Autodesk Inventor part; units mm, degrees
ref_plane "YZ Plane" through (0, 0, 0) normal (1, 0, 0) x (0, 1, 0)
ref_plane "XZ Plane" through (0, 0, 0) normal (0, 1, 0) x (-1, 0, 0)
ref_plane "XY Plane" through (0, 0, 0) normal (0, 0, 1) x (1, 0, 0)
sketch "Sketch1" plane through (0, 0, 0) normal (0, 1, 0) x (-1, 0, 0)
  line L0 (10, 67.88) -> (-10, 67.88)
  line L1 (-10, 67.88) -> (-10, -10)
  line L2 (-10, -10) -> (10, -10)
  line L3 (10, -10) -> (10, 67.88)
  point P0 (0, 0)
  dimension "d0" = 20
  dimension "d1" = 77.88
extrude "Extrusion1" add sketch "Sketch1" along normal blind 2
sketch "Sketch2" plane through (0, 2, 0) normal (0, 1, 0) x (1, 0, 0)
  line L0 (-10, -67.88) -> (10, -67.88)
  line L1 (0, -67.88) -> (-6.35, -67.88)
  line L2 (-6.35, -56.98) -> (6.35, -56.98)
  line L3 (6.35, -67.88) -> (0, -67.88)
  line L4 (10, 10) -> (-10, 10)
  line L5 (-6.35, -0.9) -> (6.35, -0.9)
  line L6 (-6.35, 10) -> (6.35, 10)
  line L7 (-6.35, -67.88) -> (-10, -67.88)
  line L8 (-10, 10) -> (-10, -67.88)
  line L9 (-10, -56.98) -> (-6.35, -56.98)
  line L10 (6.35, -67.88) -> (10, -67.88)
  line L11 (10, -67.88) -> (10, 10)
  line L12 (10, -56.98) -> (6.35, -56.98)
  line L13 (6.35, -0.9) -> (10, -0.9)
  line L14 (10, 10) -> (6.35, 10)
  line L15 (10, -0.9) -> (10, 10)
  line L16 (10, -67.88) -> (10, -56.98)
  line L17 (-10, -67.88) -> (-10, -56.98)
  line L18 (-6.35, -0.9) -> (-10, -0.9)
  line L19 (-10, -0.9) -> (-10, 10)
  line L20 (-10, 10) -> (-6.35, 10)
  point P0 (0, 0)
  dimension "d4" = 6.35
  dimension "d5" = 10.9
  dimension "d6" = 12.7
  dimension "d7" = 10.9
extrude "Extrusion2" add sketch "Sketch2" along normal blind 33.3354 contours L8 L9 L2 L12 L11 L0 | L8 L4 L11 L13 L5 L18
sketch "Sketch9" plane through (-10, 0, 67.88) normal (0, 0, 1) x (1, 0, 0)
  arc A0 (15.084, 27.3223) -> (4.684, 27.3223) centre (9.884, 27.3223) ccw
  line L0 (15.084, 20.9249) -> (15.084, 27.3223)
  line L1 (4.684, 26.1247) -> (4.684, 27.3223)
  arc A1 (15.084, 27.3223) -> (4.684, 27.3223) centre (9.884, 27.3223) ccw
  line L2 (4.684, 27.3223) -> (4.684, 20.9247)
  line L3 (9.8827, 5.3222) -> (-0.0013, 5.3222)
  line L4 (-0.0013, 15.726) -> (-0.0013, 5.3222)
  line L5 (4.684, 20.9247) -> (4.684, 15.726)
  line L6 (15.084, 20.9249) -> (15.0853, 10.5254)
  arc A2 (15.084, 20.9249) -> (15.084, 20.9251) centre (9.884, 20.9243) ccw
  line L7 (4.684, 15.726) -> (-0.0013, 15.726)
  arc A3 (9.8827, 5.3222) -> (15.0853, 10.5254) centre (9.8827, 10.5248) ccw
  line L8 (0, 35.3354) -> (20, 35.3354)
  line L9 (0, 0) -> (0, 35.3354)
  line L10 (20, 0) -> (20, 35.3354)
  point P0 (10, 0)
  point P1 (9.884, 32.5223)
  point P2 (10, 35.3354)
  point P3 (9.884, 32.5223)
  point P4 (4.9407, 5.3222)
  point P5 (2.3413, 15.726)
  point P6 (4.684, 24.1235)
  point P7 (15.084, 24.1236)
  dimension "d76" = 2.8131
  dimension "d77" = 27.2001
  dimension "d78" = 10.4039
  dimension "d79" = 10.4
  dimension "d80" = 4.684
  dimension "d81" = 4.916
fillet "Fillet4" radius 10 4 edges at (10, 35.3354, 62.43) (-10, 35.3354, 62.43) (-10, 35.3354, -4.55) (10, 35.3354, -4.55)
sketch "Sketch10" plane through (0, 2, 0) normal (0, 1, 0) x (1, 0, 0)
  line L0 (10, -67.88) -> (-10, -67.88)
  line L1 (-10, 10) -> (10, 10)
  line L2 (10, -56.98) -> (10, -0.9)
  line L3 (-10, -0.9) -> (-10, -56.98)
  line L4 (10, -28.94) -> (-10, -28.94)
  circle A0 centre (0, -28.94) radius 2.125
  point P0 (0, 0)
  dimension "d53" = 77.88
  dimension "d54" = 4.25
extrude "Extrusion10" cut sketch "Sketch10" against normal blind 2
extrude "Extrusion11" cut sketch "Sketch9" against normal through all
sketch "Sketch11" plane through (10, 0, 67.88) normal (1, 0, 0) x (0, 0, -1)
  line L0 (0, 0) -> (0, 5.3222)
  line L1 (77.88, 15.726) -> (77.88, 25.3354)
  line L2 (0, 0) -> (77.88, 0)
  line L3 (77.88, 0) -> (77.88, 25.3354)
  line L4 (77.88, 25.3354) -> (0, 25.3354)
  line L5 (0, 25.3354) -> (0, 0)
  point P0 (67.88, 0)
extrude "Extrusion12" add sketch "Sketch11" along normal blind 2
sketch "Sketch12" plane through (12, 0, 67.88) normal (1, 0, 0) x (0, 0, -1)
  line L0 (10.9, 25.3354) -> (0, 25.3354)
  line L1 (77.88, 15.726) -> (77.88, 25.3354)
  line L2 (0, 25.3354) -> (77.88, 25.3354)
  line L3 (77.88, 25.3354) -> (0, 25.3354)
  line L4 (38.94, 25.3354) -> (64.34, 25.3354)
  line L5 (38.94, 25.3354) -> (13.54, 25.3354)
  line L6 (77.88, 0) -> (0, 0)
  line L7 (13.54, 25.3354) -> (64.34, 25.3354)
  line L8 (64.34, 25.3354) -> (64.34, 0)
  line L9 (64.34, 0) -> (13.54, 0)
  line L10 (13.54, 0) -> (13.54, 25.3354)
  line L11 (13.54, 0) -> (31.84, 0)
  line L12 (31.84, 0) -> (31.84, 5)
  arc A0 (33.34, 21.3354) -> (30.34, 21.3354) centre (31.84, 21.3354) ccw
  arc A1 (30.34, 5) -> (33.34, 5) centre (31.84, 5) ccw
  line L13 (30.34, 21.3354) -> (30.34, 5)
  line L14 (33.34, 21.3354) -> (33.34, 5)
  line L15 (31.84, 21.3354) -> (13.54, 21.3354)
  point P0 (67.88, 0)
  dimension "d65" = 25.4
  dimension "d66" = 25.4
  dimension "d67" = 50.8
  dimension "d68" = 18.3
  dimension "d69" = 5
  dimension "d71" = 3
  dimension "d72" = 3
  dimension "d75" = 18.3
  dimension "d82" = 4
extrude "Extrusion13" cut sketch "Sketch12" against normal blind 2 contours A0 L14 A1 L13
sketch "Sketch14" plane through (-0.116, 27.3223, 67.88) normal (0, 0, 1) x (1, 0, 0)
  arc A0 (10.116, -1.9869) -> (-9.884, -1.9869) centre (0.116, -1.9869) ccw
  line L0 (12.116, 8.0131) -> (12.116, -1.9869)
  line L1 (12.116, 8.0131) -> (12.116, 10.0131)
  line L2 (12.116, 10.0131) -> (0.116, 10.0131)
  line L3 (0.116, 10.0131) -> (0.116, 8.0131)
  arc A1 (10.116, -1.9869) -> (-9.884, -1.9869) centre (0.116, -1.9869) ccw
  arc A2 (10.116, -1.9869) -> (0.116, 8.0131) centre (0.116, -1.9869) ccw
  line L4 (10.116, -1.9869) -> (12.116, -1.9869)
  line L5 (0.116, 8.0131) -> (0.116, 10.0131)
  line L6 (0.116, 10.0131) -> (12.116, 10.0131)
  line L7 (12.116, -1.9869) -> (12.116, 10.0131)
  point P0 (0.116, -27.3223)
  dimension "d83" = 2
extrude "Extrusion14" add sketch "Sketch14" against normal up to surface (77.88 mm away)
sketch "Sketch15" plane through (0, 37.3354, 67.88) normal (0, 1, 0) x (1, 0, 0)
  line L0 (0, 10.9) -> (0, 66.98)
  line L1 (-10, 10.9) -> (10, 10.9)
  line L2 (0, 66.98) -> (10, 66.98)
  line L3 (10, 66.98) -> (10, 10.9)
  line L4 (10, 10.9) -> (0, 10.9)
  line L5 (0, 10.9) -> (0, 66.98)
  point P0 (0, 67.88)
extrude "Extrusion15" cut sketch "Sketch15" against normal up to next
sketch "Sketch16" plane through (12, 0, 67.88) normal (1, 0, 0) x (0, 0, -1)
  arc A0 (33.34, 21.3354) -> (30.34, 21.3354) centre (31.84, 21.3354) ccw
  line L0 (66.98, 37.3354) -> (10.9, 37.3354)
  arc A1 (33.34, 33.3354) -> (30.34, 33.3354) centre (31.84, 33.3354) ccw
  line L1 (30.34, 33.3354) -> (30.34, 21.3354)
  line L2 (33.34, 33.3354) -> (33.34, 21.3354)
  arc A2 (30.34, 21.3354) -> (33.34, 21.3354) centre (31.84, 21.3354) ccw
  arc A3 (33.34, 33.3354) -> (30.34, 33.3354) centre (31.84, 33.3354) ccw
  point P0 (67.88, 0)
  dimension "d89" = 3
extrude "Extrusion16" cut sketch "Sketch16" against normal blind 2 contours A0 L1 A1 L2
properties part number "6 Backet Adjustment 3.0 short"
The listing builds one solid part. Answer for the finished solid, in the listing's coordinates (mm). A direction names the side the tool comes from. Coordinates: 2 decimals unless noted, no trailing zeros. Write each loop counter-clockwise with the first axis right and the second up, starting at its lowest first coordinate (ties: lowest second). Pieces come first, ordered by that corner, then holes. Notation, with made-up numbers: M 28.25,87.25 L 70.25,87.25 A25 ccw 70.25,122.25 Z; hole C 18.25,-20.75 d9. An arc over 180 degrees is marked long. Put each result on its own line as item: value. Start each with the question number.
1. Which of the six approach directions +Z, -Z, +X, -X, +Y, -Y give full straight-line access (tool end or side, diameter ignored) to faces 1 (the flat face through (7, 19, 0.9)), 2 (the flat face through (0, 36, -4)), 3 (the flat face through (-5.316, 21, -4)), 4 (the flat face through (-8, 15.726, 63))?
2. A cutting plane is placed at C-C on x = 3.5. Write down the section's boundary in (y, z).
3. A cutting plane is placed at B-B on y = 22. Write down the section's boundary in (x, z).
4. Flat-ended cylindrical pins translate along their axes: P1, Ø10, axis at x = 2.5, z = 2, coming from the -Y side; P2, Ø5, axis at x = -4, z = 64, coming from the +Y side; P3, Ø3, axis at y = 6, z = 6.5, coming from the -X side; P4, Ø2, axis at y = 36.5, z = 62.5, coming from the -X side. Find the tip coordinate at first contact, or state that the pin passes through.
5. For a pull along Z with two mould halves and no side action, classify faces 5 (the flat face through (6, 18, 67.88)), 6 (the flat face through (-5, 5.322, -4)), 7 (the cylindrical face through (-0.277, 1.014, 26.833)) as pulls with the +Z half, pulls with the -Z half, needs draft (parallel to the pull), parting line crosses it, or undercut.
6. A cutting plane is placed at D-D on z = 7. Write down the section's boundary in (x, y), then the cut area to 3 significant figures.
7. A cutting plane is placed at A-A on z = 36.04. Write down the section's boundary in (x, y).
8. Consider line 1 (Z direction, x = 7.75, y = 12.5); line 2 (X direction, y = 0.65, z = 28.94) (3 decimals); line 3 (Z direction, x = 0, y = 0.8) (3 decimals). Determine where each line is inside the solid, lowest interval first. Write a range as from..to.
Resolved:
1. face 1: -X, +Y
1. face 2: +Z, -Z, -X, +Y
1. face 3: +Z, -Z
1. face 4: +Z, -Z, -X
2. outline: M 0,-10 L 6.79,-10 L 6.79,0.9 L 2,0.9 L 2,56.98 L 6.79,56.98 L 6.79,67.88 L 0,67.88 Z; M 31.06,-10 L 37.34,-10 L 37.34,0.9 L 31.06,0.9 Z; M 31.06,56.98 L 37.34,56.98 L 37.34,67.88 L 31.06,67.88 Z
3. outline: M -10,-10 L -5.32,-10 L -5.32,0.9 L -10,0.9 Z; M -10,56.98 L -5.32,56.98 L -5.32,67.88 L -10,67.88 Z; M 5.08,-10 L 12,-10 L 12,34.54 L 10,34.54 L 10,0.9 L 5.08,0.9 Z; M 5.08,56.98 L 10,56.98 L 10,37.54 L 12,37.54 L 12,67.88 L 5.08,67.88 Z
4. P1: stops at y = 0
4. P2: stops at y = 35.22
4. P3: stops at x = 10
4. P4: stops at x = 0
5. face 5: pulls with the +Z half
5. face 6: needs draft
5. face 7: undercut
6. outline: M -10,0 L 12,0 L 12,37.34 L 10,37.34 L 10,2 L -10,2 Z
6. area: 115 mm2
7. outline: M -10,0 L 12,0 L 12,3.5 L 10,3.5 L 10,2 L -10,2 Z; M 10,34.84 L 12,34.84 L 12,37.34 L 10,37.34 Z
8. line 1: z = -10..0.9, 56.98..67.88
8. line 2: x = -10..-2.125, 2.125..12
8. line 3: z = -10..26.815, 31.065..67.88
